from build123d import *

# Parameters (mm, degrees)
SKETCH1_W           = 50
SKETCH1_H           = 80
BOSS_EXTRUDE1_DEPTH = 3
SKETCH2_R           = 1.5
SKETCH2_R_2         = 12.5
CUT_EXTRUDE1_DEPTH  = 48.265209192
FILLET1_R           = 5
CUT_EXTRUDE2_DEPTH  = 48.265209192


with BuildPart() as part:
    # Sketch1 → Boss-Extrude1 (new body)
    with BuildSketch(Plane(origin=(0, 0, 0), x_dir=(1, 0, 0), z_dir=(0, 1, 0))):
        Rectangle(SKETCH1_W, SKETCH1_H)
    extrude(amount=BOSS_EXTRUDE1_DEPTH)

    # Sketch2 → Cut-Extrude1 (cut, through all)
    with BuildSketch(Plane(origin=(0, 3, 0), x_dir=(1, 0, 0), z_dir=(0, 1, 0))):
        with Locations(Location((15.5, 32.5, 0), (0, 0, 270))):
            Circle(SKETCH2_R)
        with Locations(Location((-15.5, 32.5, 0), (0, 0, 270))):
            Circle(SKETCH2_R)
        with Locations(Location((-15.5, 1.5, 0), (0, 0, 270))):
            Circle(SKETCH2_R)
        with Locations(Location((15.5, 1.5, 0), (0, 0, 270))):
            Circle(SKETCH2_R)
        with Locations(Location((0, 17, 0), (0, 0, 270))):
            Circle(SKETCH2_R_2)
        with BuildLine():
            Line((-15, -28), (15, -28))
            ThreePointArc((15, -28), (17, -30), (15, -32))
            Line((15, -32), (-15, -32))
            ThreePointArc((-15, -32), (-17, -30), (-15, -28))
        make_face()
    extrude(amount=-CUT_EXTRUDE1_DEPTH, mode=Mode.SUBTRACT)

    # Fillet1
    fillet1_edges = [part.edges().sort_by_distance(p)[0] for p in [
        (-25, 1.5, -40),
        (25, 1.5, -40),
        (25, 1.5, 40),
        (-25, 1.5, 40),
    ]]
    fillet(fillet1_edges, radius=FILLET1_R)

    # Sketch3 → Cut-Extrude2 (cut, through all)
    with BuildSketch(Plane(origin=(0, 3, 0), x_dir=(1, 0, 0), z_dir=(0, 1, 0))):
        with BuildLine():
            Line((22.5, -10), (22.5, -16))
            ThreePointArc((22.5, -16), (20, -18.5), (17.5, -16))
            Line((17.5, -16), (17.5, -10))
            ThreePointArc((17.5, -10), (20, -7.5), (22.5, -10))
        make_face()
        with BuildLine():
            Line((-22.5, -10), (-22.5, -16))
            ThreePointArc((-22.5, -16), (-20, -18.5), (-17.5, -16))
            Line((-17.5, -16), (-17.5, -10))
            ThreePointArc((-17.5, -10), (-20, -7.5), (-22.5, -10))
        make_face()
    extrude(amount=-CUT_EXTRUDE2_DEPTH, mode=Mode.SUBTRACT)


solid = part.part
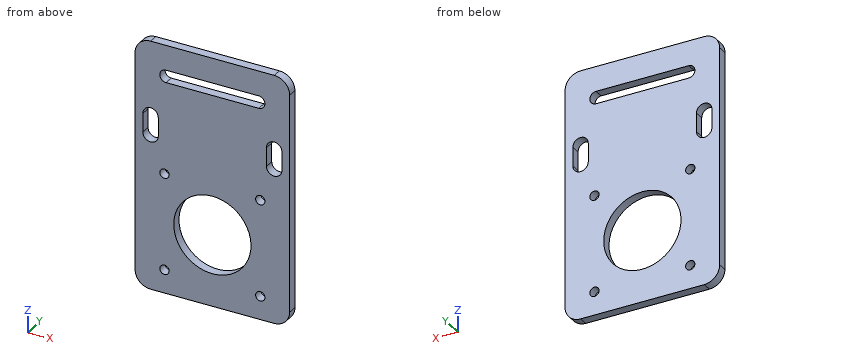
Read the model definition and answer for the solid it produces. Units are mm, in the model's axes. Coordinates: 2 decimals unless noted, no trailing zeros. Loops run counter-clockwise (first coordinate to the right, second up) from the corner with the lowest first, then second, coordinate; pieces in that order, holes last. Notation, with made-up numbers: (74.5, 38.5) - (111.5, 38.5) arc R27 ccw to (111.5, 71.5) - close; hole circle Ø10 at (52.25, 54). An arc over 180 degrees is marked (long way). Answer in a Markdown table with one row per item.
Q1. Straight lines are drawn through the part: line 1 along X through (y, z) = (1.7, -1.5); line 2 along Z through (x, y) = (-6, 1.45); line 3 along X through (y, z) = (0.95, -17). For each, find the intervals that lie inside material, in ascending order. Write a range as [from, to].
Here are the results:
| item | result |
|---|---|
| line 1 | x = [-25, -17], [-14, 14], [17, 25] |
| line 2 | z = [-40, -27.97], [-6.03, 28], [32, 40] |
| line 3 | x = [-25, -12.5], [12.5, 25] |
Q2. Find section C-C on y = 1.25. Count the separate pieces of the cut face and the enclosed holes in it, plus the area to 3 significant figures.
Here are the results:
| item | result |
|---|---|
| separate pieces | 1 |
| enclosed holes | 8 |
| area | 3,230 mm^2 |
Q3. Find section B-B on z = -32.5. Write down the section's boundary in (x, y), plus the area to 3 significant figures.
Here are the results:
| item | result |
|---|---|
| outline | (-25, 0) - (-17, 0) - (-17, 3) - (-25, 3) - close; (-14, 0) - (14, 0) - (14, 3) - (-14, 3) - close; (17, 0) - (25, 0) - (25, 3) - (17, 3) - close |
| area | 132 mm^2 |
Q4. Find section D-D on z = 30. Write down the section's boundary in (x, y), plus the area to 3 significant figures.
Here are the results:
| item | result |
|---|---|
| outline | (-25, 0) - (-17, 0) - (-17, 3) - (-25, 3) - close; (17, 0) - (25, 0) - (25, 3) - (17, 3) - close |
| area | 48.0 mm^2 |
Q5. Find section A-A on x = 0. Write down the section's boundary in (y, z), plus the area to 3 significant figures.
Here are the results:
| item | result |
|---|---|
| outline | (0, -40) - (3, -40) - (3, -29.5) - (0, -29.5) - close; (0, -4.5) - (3, -4.5) - (3, 28) - (0, 28) - close; (0, 32) - (3, 32) - (3, 40) - (0, 40) - close |
| area | 153 mm^2 |
